Verification items for this drawing (mm, ordinates from the low corner). A direction names the side the tool comes from. Give positions to 0.01 mm unless a question says otherwise; leave off trailing zeros. Order: outer loops, then holes, each group sorted by start corner. A loop starts at its lowest first (then second) coordinate and runs counter-clockwise, first axis right, second up.
(1) Mould release check, pull along Y, two halves, no side actions. Record for the marked faces 1, 2, 3 and 4: pulls with the +Y half, pulls with the -Y half, needs draft (parallel to the pull), parting line crosses it, or undercut.
(2) Sectioned sample at C-C on y = 30. Record the cut outline in (x, z).
(3) Access from +Z, -Z, +X, -X, +Y, -Y to the whole of each face (thin tool, end or side, straight path). Record for the marked faces 5 and 6.
(4) Sectioned sample at B-B on z = 25.75. Record the cut outline in (x, y), plus the area to 3 significant figures.
(5) Sectioned sample at A-A on x = 59.5. Record the cut outline in (y, z).
(6) Sectioned sample at D-D on x = 73. Record the cut outline in (y, z), plus the area to 3 significant figures.
(7) Gauge pin test, flat end, axial feed: pin 1 (1 mm diameter, centred on x = 33.5, y = 23.5, fed in from +Z). Record the tip position at first contact, or that the pin passes through.
(8) Scan lines: L1, parallel to X at y = 16.5, z = 23.5; L2, parallel to Y at x = 10, z = 6.5; L3, parallel to Z at x = 84, y = 38. Record each from-to range of solid material in increasing order.
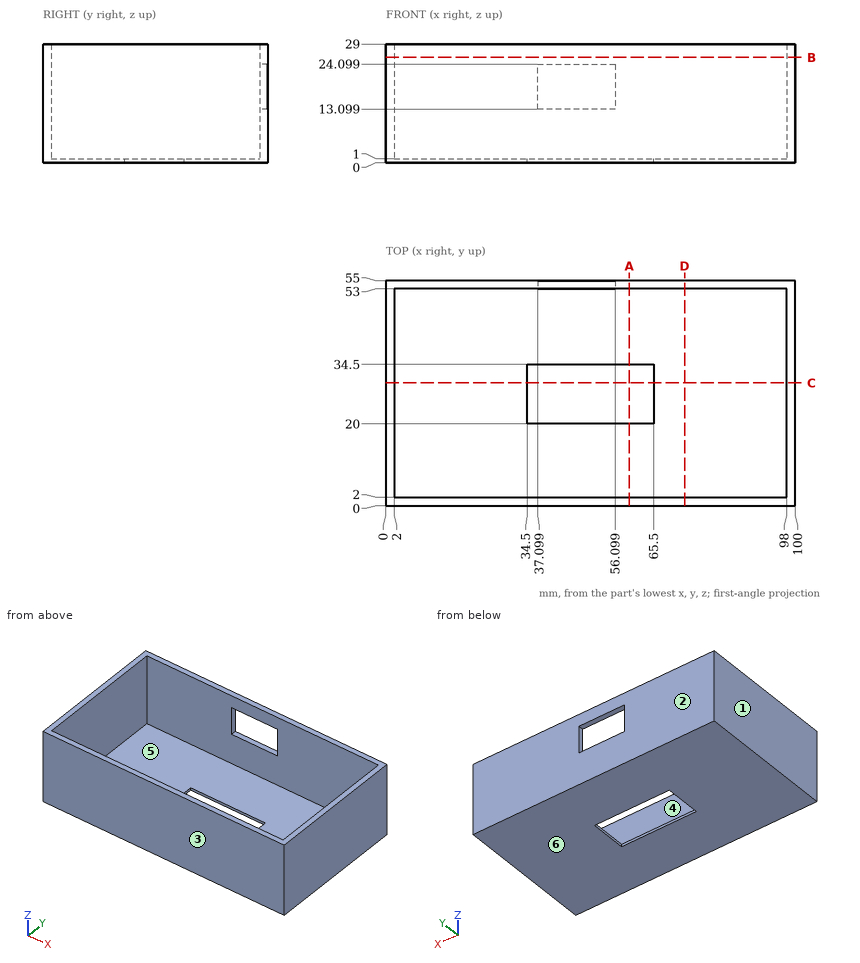
Ans:
1. face 1: needs draft
1. face 2: pulls with the +Y half
1. face 3: pulls with the -Y half
1. face 4: undercut
2. outline: (0, 0) - (34.5, 0) - (34.5, 1) - (2, 1) - (2, 29) - (0, 29) - close; (65.5, 0) - (100, 0) - (100, 29) - (98, 29) - (98, 1) - (65.5, 1) - close
3. face 5: +Z
3. face 6: -Z, +X, -X, +Y, -Y
4. outline: (0, 0) - (100, 0) - (100, 55) - (0, 55) - close; hole (2, 2) - (98, 2) - (98, 53) - (2, 53) - close
4. area: 604 mm2
5. outline: (0, 0) - (20, 0) - (20, 1) - (2, 1) - (2, 29) - (0, 29) - close; (34.5, 0) - (55, 0) - (55, 29) - (53, 29) - (53, 1) - (34.5, 1) - close
6. outline: (0, 0) - (55, 0) - (55, 29) - (53, 29) - (53, 1) - (2, 1) - (2, 29) - (0, 29) - close
6. area: 167 mm2
7. pin 1: stops at z = 1
8. L1: x = 0 to 2, 98 to 100
8. L2: y = 0 to 2, 53 to 55
8. L3: z = 0 to 1
